For this review, take the finished solid that the model builds, in its own axes (mm). A direction names the side the tool comes from. Round coordinates to 2 decimals unless told otherwise and drop trailing zeros. Order: outer loops, then holes, each group sorted by start corner. A loop starts at its lowest first (then second) coordinate and runs counter-clockwise, first axis right, second up. Notation, with made-up numbers: M -3.75,-21.75 L 11.25,-21.75 A17 cw 11.25,3.25 Z; hole C -18.75,72 d4. An arc over 180 degrees is marked long. Put each result on its own line as item: value.
from build123d import *

# Parameters (mm, degrees)
SKETCH1_R           = 11.5
SKETCH1_W           = 4
SKETCH1_H           = 4
BOSS_EXTRUDE1_DEPTH = 4
SKETCH2_R           = 2
CUT_EXTRUDE1_DEPTH  = 4


with BuildPart() as part:
    # Sketch1 → Boss-Extrude1 (new body)
    with BuildSketch(Plane.XY):
        Circle(SKETCH1_R)
        with Locations((0, 7.5)):
            Rectangle(SKETCH1_W, SKETCH1_H, mode=Mode.SUBTRACT)
        with Locations((7.5, 0)):
            Rectangle(SKETCH1_W, SKETCH1_H, mode=Mode.SUBTRACT)
        with Locations((0, -7.5)):
            Rectangle(SKETCH1_W, SKETCH1_H, mode=Mode.SUBTRACT)
        with Locations((-7.5, 0)):
            Rectangle(SKETCH1_W, SKETCH1_H, mode=Mode.SUBTRACT)
    extrude(amount=BOSS_EXTRUDE1_DEPTH)

    # Sketch2 → Cut-Extrude1 (cut)
    with BuildSketch(Plane.XY.offset(4)):
        Circle(SKETCH2_R)
    extrude(amount=-CUT_EXTRUDE1_DEPTH, mode=Mode.SUBTRACT)


solid = part.part
(1) Add section A-A on y = 0. Give the boundary of the cut face in (x, z).
A:
outline: M -11.5,0 L -9.5,0 L -9.5,4 L -11.5,4 Z; M -5.5,0 L -2,0 L -2,4 L -5.5,4 Z; M 2,0 L 5.5,0 L 5.5,4 L 2,4 Z; M 9.5,0 L 11.5,0 L 11.5,4 L 9.5,4 Z
(2) Add section D-D on x = -6.25. Give the boundary of the cut face in (y, z), then the cut area to 3 significant figures.
A:
outline: M -9.65,0 L -2,0 L -2,4 L -9.65,4 Z; M 2,0 L 9.65,0 L 9.65,4 L 2,4 Z
area: 61.2 mm2
(3) To check wall thickness, follow L1, parallel to Y at x = 0, z = 2.7; L2, parallel to X at y = -0.5, z = 2.1; L3, parallel to X at y = -8.5, z = 3.6. State the ranges of each line that lie inside material, in increasing order.
A:
L1: y = -11.5 to -9.5, -5.5 to -2, 2 to 5.5, 9.5 to 11.5
L2: x = -11.49 to -9.5, -5.5 to -1.94, 1.94 to 5.5, 9.5 to 11.49
L3: x = -7.75 to -2, 2 to 7.75
(4) For faces 1 (the face through (-0.2, -2.4, 0)), 2 (the face through (5.5, 0, 2)), list the 3-axis set-ups (+Z, -Z, +X, -X, +Y, -Y) from which the entire face can be reached by the end or side of a thin tool; tool diameter is ignored.
A:
face 1: -Z, +X, -X, +Y, -Y
face 2: +Z, -Z
(5) Insertion check: pin 1 Ø1.2 at (x, z) = (-1, 2.5) entering from -Y; pin 2 Ø1.5 at (y, z) = (3.5, 2) entering from +X; pin 3 Ø2 at (y, z) = (-7, 2.5) entering from -X. Each pin has a flat end and moves straight along its axis. Give the tip position at first contact, or say it passes through.
A:
pin 1: stops at y = -11.49
pin 2: stops at x = 11.17
pin 3: stops at x = -9.81
(6) Draft analysis for pull direction Y (two halves, no side actions). For faces 3 (the face through (-5.5, 0, 2)), 4 (the face through (-0.2, -2.4, 4)), state which applies: released by +Y, released by -Y, zero draft, split by the parting line, or undercut.
A:
face 3: undercut
face 4: zero draft
(7) Add section C-C on z = 2.4. Give the boundary of the cut face in (x, y), then the cut area to 3 significant figures.
A:
outline: C 0,0 d23; hole M -9.5,-2 L -5.5,-2 L -5.5,2 L -9.5,2 Z; hole M -2,-9.5 L 2,-9.5 L 2,-5.5 L -2,-5.5 Z; hole C 0,0 d4; hole M -2,5.5 L 2,5.5 L 2,9.5 L -2,9.5 Z; hole M 5.5,-2 L 9.5,-2 L 9.5,2 L 5.5,2 Z
area: 339 mm2
